Geometry: final body of the model. Coordinates: model frame, mm. Give positions to 0.01 mm unless a question says otherwise; leave off trailing zeros. Order: outer loops, then holes, each group sorted by start corner. A loop starts at its lowest first (then second) coordinate and runs counter-clockwise, first axis right, second up. Notation, with made-up numbers: M 66.5,-1 L 106.5,-1 A23 ccw 106.5,16 Z; hole C 40,45 d3. An arc over 180 degrees is marked long. Write item = value, one per line. Start each with the question number.
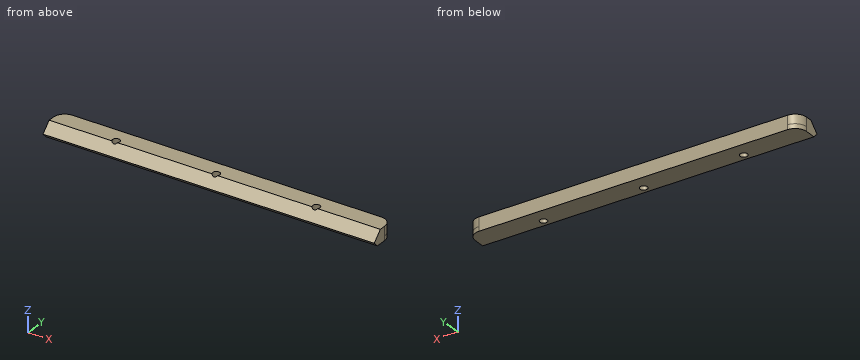
from build123d import *

# Parameters (mm, degrees)
BOSS_EXTRUDE1_DEPTH       = 36.4
FILLET3_R                 = 2.5
CUT_EXTRUDE5_DEPTH        = 72.8
BOSS_EXTRUDE2_DEPTH       = 72.8
M2X0_4_TAPPED_HOLE1_D     = 1.6
M2X0_4_TAPPED_HOLE1_DEPTH = 3.6
M2X0_4_TAPPED_HOLE1_TIP   = 0.480688495
FILLET4_R                 = 2.5


with BuildPart() as part:
    # Sketch1 → Boss-Extrude1 (new, symmetric)
    with BuildSketch(Plane(origin=(0, 0, 0), x_dir=(0, 0, -1), z_dir=(1, 0, 0))):
        Polygon((0, -3.2), (-2, -1.2), (-2, 3.2), (0, 3.2), align=None)
    extrude(amount=BOSS_EXTRUDE1_DEPTH, both=True)

    # Fillet3
    fillet3_edges = [part.edges().sort_by_distance(p)[0] for p in [
        (-36.4, 3.2, 1),
        (36.4, 3.2, 1),
    ]]
    fillet(fillet3_edges, radius=FILLET3_R)

    # Sketch5 → Cut-Extrude5 (cut)
    with BuildSketch(Plane.ZY.offset(36.4)):
        Polygon((0, -2.7), (2, -0.7), (2, -1.2), (0, -3.2), align=None)
    extrude(amount=-CUT_EXTRUDE5_DEPTH, mode=Mode.SUBTRACT)

    # Sketch7 → Boss-Extrude2 (add)
    with BuildSketch(Plane.ZY.offset(36.4)):
        Polygon((0, -2.7), (-1, -1.7), (-1, 3.2), (0, 3.2), align=None)
    extrude(amount=-BOSS_EXTRUDE2_DEPTH)

    # M2x0.4 Tapped Hole1
    with Locations(Plane.XY.offset(2)):
        with Locations((-22, -0.2), (22, -0.2), (0, -0.2)):
            Hole(M2X0_4_TAPPED_HOLE1_D / 2, depth=M2X0_4_TAPPED_HOLE1_DEPTH)
            with Locations((0, 0, -(M2X0_4_TAPPED_HOLE1_DEPTH + M2X0_4_TAPPED_HOLE1_TIP / 2))):  # 118° drill point
                Cone(0, M2X0_4_TAPPED_HOLE1_D / 2, M2X0_4_TAPPED_HOLE1_TIP, mode=Mode.SUBTRACT)

    # Fillet4
    fillet4_edges = [part.edges().sort_by_distance(p)[0] for p in [
        (-36.4, 3.2, -0.5),
        (36.4, 3.2, -0.5),
    ]]
    fillet(fillet4_edges, radius=FILLET4_R)


solid = part.part
1) Cut plane C-C (x = -3). Return loops of the section in (y, z).
2) Pin query (flat end, axial travel): pin 1 Ø2.5 at (x, y) = (-22, -0.2) entering from +Z. Return the tip coordinate at first contact, or that it passes through.
3) Cut plane B-B (z = 0.6). Return loops of the section in (x, y).
4) Ray query, L1, parallel to X at y = -0.2, z = 0.4; L2, parallel to X at y = -0.5, z = 1.7; L3, parallel to Y at x = 21.5, z = 1.45. Return the intervals inside material, ascending.
5) Cut plane A-A (x = 22). Return loops of the section in (y, z).
Reply:
q1.outline = M -2.7,0 L -1.7,-1 L 3.2,-1 L 3.2,2 L -0.7,2 Z
q2.pin_1 = 2
q3.outline = M -36.4,-2.1 L 36.4,-2.1 L 36.4,0.7 A2.5 ccw 33.9,3.2 L -33.9,3.2 A2.5 ccw -36.4,0.7 Z; hole C -22,-0.2 d1.6; hole C 0,-0.2 d1.6; hole C 22,-0.2 d1.6
q4.L1 = -36.4 to -22.8, -21.2 to -0.8, 0.8 to 21.2, 22.8 to 36.4
q4.L2 = -36.4 to -22.74, -21.26 to -0.74, 0.74 to 21.26, 22.74 to 36.4
q4.L3 = -1.25 to -0.82, 0.42 to 3.2
q5.outline = M -2.7,0 L -1.7,-1 L -1,-1 L -1,1.7 Z; M 0.6,-1 L 3.2,-1 L 3.2,2 L 0.6,2 Z
